Build history of the part. All positions in model axes, mm. Face numbers are marked on the shaded views. A direction names the side the tool comes from. Give positions to 0.01 mm unless a question says otherwise; leave off trailing zeros. Write each loop counter-clockwise with the first axis right and the second up, starting at its lowest first coordinate (ties: lowest second). Pieces come first, ordered by that corner, then holes. Notation, with made-up numbers: (8, 28.5) -> (20, 28.5) arc R9 ccw to (20, 40.5) -> close; hole circle Ø2 at (-3.75, -21). An arc over 180 degrees is marked (long way). Write item = value, one per line. Start each with the question number.
Q1. Wall check: line 1 (X direction, y = 11.5, z = -0.5); line 2 (Z direction, x = -32, y = 15.75); line 3 (X direction, y = 24, z = 16). Give the ranges that are in metal, low to high.
Q2. Saw through at B-B, the plane z = -6. List the corners of the cut face in (x, y), then the cut area to 3 significant figures.
Q3. Drop flat-ended pins along their axis: P1, Ø7.5, axis at y = 13.5, z = -6.5, coming from the -X side; P2, Ø12.5, axis at y = 12, z = 7.5, coming from the +X side; P3, Ø14, axis at x = -35, y = 9.5, coming from the +Z side; P4, Ø3.5, axis at x = -33.274, y = 6.35, coming from the +Z side. Give the stop position or say it passes through.
Q4. Saw through at A-A, the plane y = 19.05. List the corners of the cut face in (x, z).
Q5. Saw through at D-D, the plane x = -28. List the corners of the cut face in (y, z).
Q6. Tool access for the marked faces 1, 2 and 3: list every direction of +Z, -Z, +X, -X, +Y, -Y with a clear straight run to the whole face (end or side of a thin tool).
Q7. Mould opens along X. For the marked faces 4, 5, 6 and 7 say: pulls with the +X half, pulls with the -X half, needs draft (parallel to the pull), parting line crosses it, or undercut.
Q8. Saw through at C-C, the plane y = 12.7. List the corners of the cut face in (x, z), then the cut area to 3 significant figures.
from build123d import *

# Parameters (mm, degrees)
BOSS_EXTRUDE1_DEPTH    = 25.4
SKETCH2_R              = 2.032
CUT_EXTRUDE1_DEPTH     = 62.309334692
F_10_32_TAPPED_HOLE1_D = 4.0386


with BuildPart() as part:
    # Sketch1 → Boss-Extrude1 (new body)
    with BuildSketch(Plane(origin=(0, 0, 0), x_dir=(1, 0, 0), z_dir=(0, 1, 0))):
        with BuildLine():
            Line((-20.574, -9.652129604), (-4.162019583, -14.39674322))
            ThreePointArc((-4.162019583, -14.39674322), (12.103082443, -8.837647749), (12.446, 8.347796497))
            Line((12.446, 8.347796497), (12.446, 20.746712887))
            Line((12.446, 20.746712887), (31.496, 20.746712887))
            Line((31.496, 20.746712887), (31.496, 17.571712887))
            Line((31.496, 17.571712887), (18.796, 17.571712887))
            Line((18.796, 17.571712887), (18.796, -12.827129604))
            Line((18.796, -12.827129604), (18.796, -21.717129604))
            Line((18.796, -21.717129604), (-26.924, -21.717129604))
            Line((-26.924, -21.717129604), (-26.924, -12.827129604))
            Line((-26.924, -12.827129604), (-26.924, 17.571712887))
            Line((-26.924, 17.571712887), (-39.624, 17.571712887))
            Line((-39.624, 17.571712887), (-39.624, 20.746712887))
            Line((-39.624, 20.746712887), (-20.574, 20.746712887))
            Line((-20.574, 20.746712887), (-20.574, 9.652))
            Line((-20.574, 9.652), (-20.574, -9.652129604))
        make_face()
    extrude(amount=BOSS_EXTRUDE1_DEPTH)

    # Sketch2 → Cut-Extrude1 (cut, through all)
    with BuildSketch(Plane.XY.offset(-17.571712887)):
        with Locations((-33.274, 19.05)):
            Circle(SKETCH2_R)
        with Locations((-33.274, 6.35)):
            Circle(SKETCH2_R)
        with Locations((25.146, 19.05)):
            Circle(SKETCH2_R)
        with Locations((25.146, 6.35)):
            Circle(SKETCH2_R)
    extrude(amount=-CUT_EXTRUDE1_DEPTH, mode=Mode.SUBTRACT)

    # #10-32 Tapped Hole1 (through all)
    with Locations(Plane.XY.offset(21.717129604)):
        with Locations((-4.064, 12.7)):
            Hole(F_10_32_TAPPED_HOLE1_D / 2)


solid = part.part
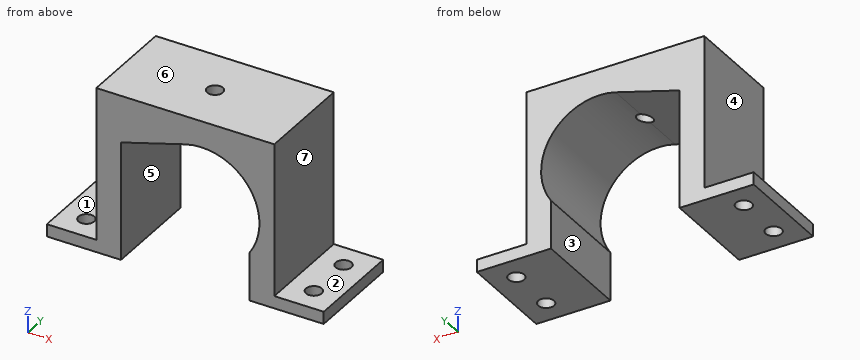
Report:
q1.line_1 = -26.92 to -20.57, 14.98 to 18.8
q1.line_2 = -20.75 to -17.57
q1.line_3 = -26.92 to 18.8
q2.outline = (-26.92, 0) -> (-20.57, 0) -> (-20.57, 25.4) -> (-26.92, 25.4) -> close; (13.73, 0) -> (18.8, 0) -> (18.8, 25.4) -> (13.73, 25.4) -> close
q2.area = 290 mm2
q3.P1 = -26.92
q3.P2 = 18.8
q3.P3 = -17.57
q3.P4 = through
q4.outline = (-39.62, -20.75) -> (-35.31, -20.75) -> (-35.31, -17.57) -> (-39.62, -17.57) -> close; (-31.24, -20.75) -> (-20.57, -20.75) -> (-20.57, 9.65) -> (-4.16, 14.4) arc R14.99 cw to (12.45, -8.35) -> (12.45, -20.75) -> (23.11, -20.75) -> (23.11, -17.57) -> (18.8, -17.57) -> (18.8, 21.72) -> (-26.92, 21.72) -> (-26.92, -17.57) -> (-31.24, -17.57) -> close; (27.18, -20.75) -> (31.5, -20.75) -> (31.5, -17.57) -> (27.18, -17.57) -> close
q5.outline = (0, -20.75) -> (25.4, -20.75) -> (25.4, -17.57) -> (0, -17.57) -> close
q6.face_1 = +Z, -X, +Y, -Y
q6.face_2 = +Z, +X, +Y, -Y
q6.face_3 = -Z, +Y, -Y
q7.face_4 = pulls with the -X half
q7.face_5 = undercut
q7.face_6 = needs draft
q7.face_7 = pulls with the +X half
q8.outline = (-39.62, -20.75) -> (-20.57, -20.75) -> (-20.57, 9.65) -> (-6.08, 13.84) -> (-6.08, 21.72) -> (-26.92, 21.72) -> (-26.92, -17.57) -> (-39.62, -17.57) -> close; (-2.04, 14.85) arc R14.99 cw to (12.45, -8.35) -> (12.45, -20.75) -> (31.5, -20.75) -> (31.5, -17.57) -> (18.8, -17.57) -> (18.8, 21.72) -> (-2.04, 21.72) -> close
q8.area = 858 mm2
